from build123d import *

# Parameters (mm, degrees)
SKETCH1_W           = 38.1
SKETCH1_H           = 38.1
BOSS_EXTRUDE1_DEPTH = 6.35
SKETCH2_W           = 33.02
SKETCH2_H           = 33.02
CUT_EXTRUDE1_DEPTH  = 5.08
SKETCH5_R           = 10.755
CUT_EXTRUDE5_DEPTH  = 5.08
FILLET7_R           = 2.032
FILLET8_R           = 2.032


with BuildPart() as part:
    # Sketch1 → Boss-Extrude1 (new body)
    with BuildSketch(Plane(origin=(0, 0, 0), x_dir=(1, 0, 0), z_dir=(0, 1, 0))):
        Rectangle(SKETCH1_W, SKETCH1_H)
    extrude(amount=BOSS_EXTRUDE1_DEPTH)

    # Sketch2 → Cut-Extrude1 (cut)
    with BuildSketch(Plane(origin=(0, 6.35, 0), x_dir=(1, 0, 0), z_dir=(0, 1, 0))):
        Polygon((-16.51, 19.05), (-19.05, 19.05), (-19.05, 16.51), (-19.05, -16.51), (-19.05, -19.05), (-16.51, -19.05), (16.51, -19.05), (19.05, -19.05), (19.05, -16.51), (19.05, 16.51), (19.05, 19.05), (16.51, 19.05), align=None)
        Rectangle(SKETCH2_W, SKETCH2_H, mode=Mode.SUBTRACT)
    extrude(amount=-CUT_EXTRUDE1_DEPTH, mode=Mode.SUBTRACT)

    # Sketch5 → Cut-Extrude5 (cut)
    with BuildSketch(Plane.XZ):
        with Locations(Location((0, 0, 0), (0, 0, 270))):
            Circle(SKETCH5_R)
    extrude(amount=-CUT_EXTRUDE5_DEPTH, mode=Mode.SUBTRACT)

    # Fillet7
    fillet7_edges = [part.edges().sort_by_distance(p)[0] for p in [
        (0, 5.08, 10.755),
    ]]
    fillet(fillet7_edges, radius=FILLET7_R)

    # Fillet8
    fillet8_edges = [part.edges().sort_by_distance(p)[0] for p in [
        (0, 0, 10.755),
    ]]
    fillet(fillet8_edges, radius=FILLET8_R)


solid = part.part
Model file for the job. Use its own axes, mm. A direction names the side the tool comes from. Give positions to 0.01 mm unless a question says otherwise; leave off trailing zeros. Write each loop counter-clockwise with the first axis right and the second up, starting at its lowest first coordinate (ties: lowest second). Pieces come first, ordered by that corner, then holes. Notation, with made-up numbers: (-5.5, 9) - (43.5, 9) arc R22 ccw to (43.5, 29) - close; hole circle Ø4 at (85, 41). An arc over 180 degrees is marked (long way). Answer as CSV lines item,"result".
1. 3-axis set-ups, long thin cutter, end or side, ignore diameter. For faces 4 (the face through (0, 4, -16.51)), 5 (the face through (0, 5.08, 0)), 6 (the face through (0, 4, 16.51)): which of +Z, -Z, +X, -X, +Y, -Y reach the whole face in a straight line?
Responses:
face 4,"-Z, +X, -X, +Y"
face 5,"-Y"
face 6,"+Z, +X, -X, +Y"
2. Band-saw the part on A-A (x = 0). Write the cut outline in (y, z) (3 decimals).
Responses:
outline,"(0, -19.05) - (1.27, -19.05) - (1.27, -16.51) - (6.35, -16.51) - (6.35, 16.51) - (1.27, 16.51) - (1.27, 19.05) - (0, 19.05) - (0, 12.787) arc R2.032 ccw to (2.032, 10.755) - (3.048, 10.755) arc R2.032 cw to (5.08, 8.723) - (5.08, -8.723) arc R2.032 cw to (3.048, -10.755) - (2.032, -10.755) arc R2.032 ccw to (0, -12.787) - close"
3. Two-plate mould, pull along Z, no slides. Class faces 1 (the face through (0, 1, 19.05)), 2 (the face through (16.51, 4, 0)), 3 (the face through (-6.544, 2.533, 8.535)): +Z half, -Z half, draft (parallel to the pull), parting line (faces both ways), or undercut.
Responses:
face 1,"+Z half"
face 2,"draft"
face 3,"undercut"
4. Drill centre lines: L1, parallel to X at y = 2.6, z = 0 (3 decimals); L2, parallel to Z at x = 4.5, y = 2.75; L3, parallel to X at y = 2.5, z = 8. Where is each one in solid material? Low to high. Write a range as [from, to].
Responses:
L1,"x = [-16.51, -10.755], [10.755, 16.51]"
L2,"z = [-16.51, -9.77], [9.77, 16.51]"
L3,"x = [-16.51, -7.19], [7.19, 16.51]"
5. Band-saw the part on B-B (z = 0). Write the cut outline in (x, y) (3 decimals).
Responses:
outline,"(-19.05, 0) - (-12.787, 0) arc R2.032 ccw to (-10.755, 2.032) - (-10.755, 3.048) arc R2.032 cw to (-8.723, 5.08) - (8.723, 5.08) arc R2.032 cw to (10.755, 3.048) - (10.755, 2.032) arc R2.032 ccw to (12.787, 0) - (19.05, 0) - (19.05, 1.27) - (16.51, 1.27) - (16.51, 6.35) - (-16.51, 6.35) - (-16.51, 1.27) - (-19.05, 1.27) - close"
6. Pin check, flat tips, straight feed: pin 1 (3 mm diameter, centred on y = 3, z = 3.5, fed in from +X); pin 2 (2.5 mm diameter, centred on x = -7.5, y = 3, fed in from -Z); pin 3 (5 mm diameter, centred on x = 4, z = 2, fed in from -Y). Stop position of each tip, or through.
Responses:
pin 1,"stops at x = 16.51"
pin 2,"stops at z = -16.51"
pin 3,"stops at y = 5.08"
